Work out the finished part from the listing and answer in its coordinate system (mm). A direction names the side the tool comes from. Give positions to 0.01 mm unless a question says otherwise; leave off trailing zeros. Order: outer loops, then holes, each group sorted by start corner. A loop starts at its lowest first (then second) coordinate and runs counter-clockwise, first axis right, second up. Notation, with made-up numbers: M -25,-30.75 L -9,-30.75 A18 ccw -9,-23.75 Z; hole C 75.5,89 d6. An arc over 180 degrees is marked long. One line per item, written item: value.
from build123d import *

# Parameters (mm, degrees)
F0_W     = 939.8
F0_H     = 520.7
F1_DEPTH = 50.8
F4_DEPTH = 50.8
F5_D     = 6.35
F7_R     = 3.175
F8_DEPTH = 50.8


with BuildPart() as f1:
    # F0 (on Top) → F1 (new body)
    with BuildSketch(Plane.XY):
        with Locations((469.9, 260.35)):
            Rectangle(F0_W, F0_H)
    extrude(amount=F1_DEPTH)

    # F3 (on offset) → F4 (join)
    with BuildSketch(Plane.YZ.offset(850.9)):
        with BuildLine():
            ThreePointArc((549.275, 6.35), (540.9055762724, 26.5555762724), (520.7, 34.925))
            Line((520.7, 34.925), (520.7, 6.35))
            Line((520.7, 6.35), (549.275, 6.35))
        make_face()
    extrude(amount=-F4_DEPTH)

    # F5 (through all)
    with Locations(Plane.YZ.offset(850.9)):
        with Locations((539.75, 12.7)):
            Hole(F5_D / 2)

    # F7 (on offset) → F8 (join)
    with BuildSketch(Plane(origin=(88.9, 0, 0), x_dir=(0, -1, 0), z_dir=(-1, 0, 0))):
        with BuildLine():
            ThreePointArc((-520.7, 34.925), (-540.9055762724, 26.5555762724), (-549.275, 6.35))
            Line((-549.275, 6.35), (-520.7, 6.35))
            Line((-520.7, 6.35), (-520.7, 34.925))
        make_face()
        with Locations((-539.75, 12.7)):
            Circle(F7_R, mode=Mode.SUBTRACT)
    extrude(amount=-F8_DEPTH)


solid = f1.part
(1) Which of the six approach directions +Z, -Z, +X, -X, +Y, -Y give full straight-line access (tool end or side, diameter ignored) to faces 5 (the flat face through (800.1, 532, 18)), 6 (the flat face through (88.9, 532, 18)), 7 (the flat face through (826, 535, 6.35))?
Findings:
face 5: +Z, -Z, +Y
face 6: +Z, -Z, -X, +Y
face 7: -Z, +X, -X, +Y
(2) Section A-A, the plane x = 557.5 is taken. Give the vertices of the cut face in (y, z).
Findings:
outline: M 0,0 L 520.7,0 L 520.7,50.8 L 0,50.8 Z
(3) Given P1, Ø14.5, axis at y = 541, z = 17.5, coming from the -X side; P2, Ø14.5, axis at y = 530.5, z = 19, coming from the +X side; P3, Ø8.5, axis at x = 124.5, y = 529.5, coming from the -Z side, each flat-ended and moving along its own axis, determine where each tip first touches the part or whether it passes through.
Findings:
P1: stops at x = 88.9
P2: stops at x = 850.9
P3: stops at z = 6.35
(4) Determine the mould class of faces 1 (the flat face through (850.9, 532, 18)), 2 (the flat face through (463, 0, 25)), 3 (the flat face through (463, 520.7, 25)), 4 (the flat face through (139.7, 532, 18)) for opening direction X: pulls with the +X half, pulls with the -X half, needs draft (parallel to the pull), parting line crosses it, or undercut.
Findings:
face 1: pulls with the +X half
face 2: needs draft
face 3: undercut
face 4: undercut
(5) Find the intervals of material crossed by probe 1 along Y at (x, z) = (449, 7); probe 2 along Z at (x, y) = (834, 539); probe 3 along Y at (x, z) = (120, 12), in increasing order. Write a range as from..to.
Findings:
probe 1: y = 0..520.7
probe 2: z = 6.35..9.61, 15.79..28.3
probe 3: y = 0..536.65, 542.85..548.71
